Autodesk Inventor part; units mm, degrees
ref_plane "YZ Plane" through (0, 0, 0) normal (1, 0, 0) x (0, 1, 0)
ref_plane "XZ Plane" through (0, 0, 0) normal (0, 1, 0) x (-1, 0, 0)
ref_plane "XY Plane" through (0, 0, 0) normal (0, 0, 1) x (1, 0, 0)
sketch "Sketch1" plane through (0, 0, 0) normal (0, 0, 1) x (1, 0, 0)
  line L0 (0, 0) -> (0, 32)
  line L1 (0, 32) -> (6, 32)
  line L2 (6, 32) -> (32, 6)
  line L3 (32, 6) -> (32, 0)
  line L4 (32, 0) -> (0, 0)
  dimension "d0" = 32
  dimension "d1" = 6
extrude "Extrusion1" add sketch "Sketch1" along normal mid plane 25
sketch "Sketch2" plane through (0, 32, 12.5) normal (0, 1, 0) x (1, 0, 0)
  line L0 (0, 0) -> (0, 25)
  line L1 (6, 0) -> (0, 0)
  line L2 (0, 25) -> (6, 25)
  line L3 (3, 22) -> (32, 22)
  line L4 (32, 22) -> (32, 3)
  line L5 (32, 3) -> (3, 3)
  line L6 (3, 3) -> (3, 22)
  line L7 (32, 0) -> (32, 25)
  point P0 (0, 12.5)
  dimension "d4" = 3
  dimension "d5" = 3
  dimension "d6" = 3
extrude "Extrusion2" cut sketch "Sketch2" against normal blind 29
equation "\"d5\" = d4"
equation "\"d6\" = d4"
properties part number "CornerBracket"
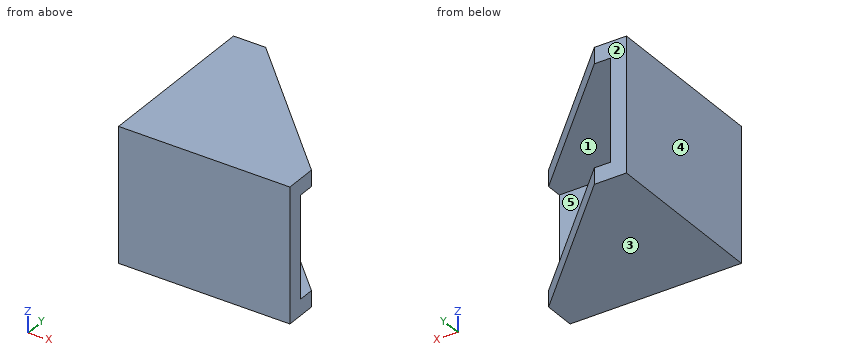
Here's how the part is built. I have some questions about the finished solid (model axes, mm). Face numbers are marked on the shaded views. A direction names the side the tool comes from. Give positions to 0.01 mm unless a question says otherwise; leave off trailing zeros. Write each loop counter-clockwise with the first axis right and the second up, starting at its lowest first coordinate (ties: lowest second). Pieces come first, ordered by that corner, then holes.
(1) Imagine slicing it at C-C, the plane z = 11.25. Write out the boundary of the cut face in (x, y), and give its area (3 significant figures).
Output values:
outline: (0, 0) - (32, 0) - (32, 6) - (6, 32) - (0, 32) - close
area: 686 mm2
(2) If I drill on L1, parallel to Z at x = 13.5, y = 14.5; L2, parallel to Y at x = 5, z = 0, over which ranges is the centre line in solid material (lowest first)?
Output values:
L1: z = -12.5 to -9.5, 9.5 to 12.5
L2: y = 0 to 3
(3) On a 3-axis mill with a long thin cutter (end or side, diameter ignored), from which of +Z, -Z, +X, -X, +Y, -Y can I reach the whole of each face in a straight line? I mean the marked faces 1 and 2. Say none if no direction works.
Output values:
face 1: +X, +Y
face 2: +Z, -Z, +X, -X, +Y
(4) Will these pins go through, and if not, where does the flat tip stop? pin 1 (8 mm diameter, centred on x = 4, z = 4.5, fed in from -Y); pin 2 (9.5 mm diameter, centred on x = 18, z = 4.5, fed in from +Y); pin 3 (3 mm diameter, centred on x = 8, z = 9.5, fed in from +Y).
Output values:
pin 1: stops at y = 0
pin 2: stops at y = 3
pin 3: stops at y = 31.5
(5) Thinking about a two-plate mould opening in Z: for the marked faces 3, 4 and 5, which applies, pulls with the +Z half, pulls with the -Z half, needs draft (parallel to the pull), parting line crosses it, or undercut?
Output values:
face 3: pulls with the -Z half
face 4: needs draft
face 5: undercut
(6) Imagine slicing it at A-A, the plane y = 10.5. Write out the boundary of the cut face in (x, z), and give its area (3 significant figures).
Output values:
outline: (0, -12.5) - (27.5, -12.5) - (27.5, -9.5) - (3, -9.5) - (3, 9.5) - (27.5, 9.5) - (27.5, 12.5) - (0, 12.5) - close
area: 222 mm2
(7) Imagine slicing it at D-D, the plane z = -8.75. Write out the boundary of the cut face in (x, y).
Output values:
outline: (0, 0) - (32, 0) - (32, 3) - (3, 3) - (3, 32) - (0, 32) - close
(8) Imagine slicing it at B-B, the plane x = 21. Write out the boundary of the cut face in (y, z), and give its area (3 significant figures).
Output values:
outline: (0, -12.5) - (17, -12.5) - (17, -9.5) - (3, -9.5) - (3, 9.5) - (17, 9.5) - (17, 12.5) - (0, 12.5) - close
area: 159 mm2
